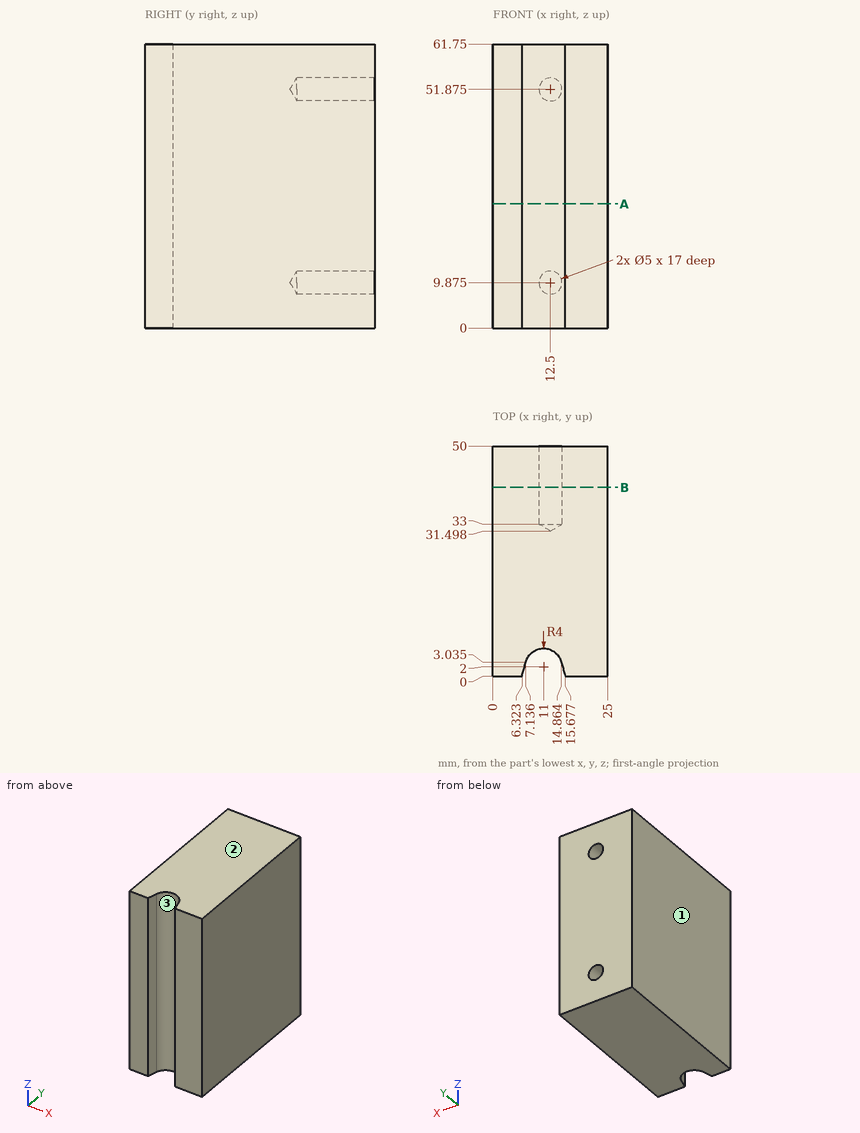
Source: three-view drawing plus pictorial views. Frame: mm from the lowest corner of the part. Give positions to 0.01 mm unless a question says otherwise; leave off trailing zeros. Order: outer loops, then holes, each group sorted by start corner. A loop starts at its lowest first (then second) coordinate and runs counter-clockwise, first axis right, second up.
1. Section A-A on z = 27. Return the cut outline in (x, y) (1 decimal), and give its area (3 significant figures).
Derived:
outline: (0, 0) - (6.3, 0) - (7.1, 3) arc R4 cw to (14.9, 3) - (15.7, 0) - (25, 0) - (25, 50) - (0, 50) - close
area: 1,210 mm2
2. Material intervals for L1, parallel to X at y = 47.5, z = 52.5; L2, parallel to Z at x = 13.5, y = 44; L3, parallel to X at y = 32.5, z = 9.5 (1 decimal), sorted ascending.
Derived:
L1: x = 0 to 10.08, 14.92 to 25
L2: z = 0 to 7.58, 12.17 to 49.58, 54.17 to 61.75
L3: x = 0 to 10.9, 14.1 to 25
3. Mould query, pull axis X, two halves, no side actions, for the marked faces 1, 2 and 3. Classes: released by +X, released by -X, zero draft, split by the parting line, or undercut.
Derived:
face 1: released by -X
face 2: zero draft
face 3: undercut
4. Section B-B on y = 41. Give the number of separate pieces and of enclosed holes in the cut face, and give its area (3 significant figures).
Derived:
separate pieces: 1
enclosed holes: 2
area: 1,500 mm2
